Geometry: see drawing. Coordinates: mm, zero at the bounding-box minimum. A direction names the side the tool comes from. Give positions to 0.01 mm unless a question says otherwise; leave off trailing zeros. Write each loop counter-clockwise with the first axis right and the second up, starting at its lowest first coordinate (ties: lowest second). Pieces come first, ordered by that corner, then holes. Notation, with made-up numbers: (78.25, -3.75) -> (130.25, -3.75) arc R20 cw to (130.25, 35.25) -> close; hole circle Ø6 at (88, 88.5). An arc over 180 degrees is marked (long way). Answer as a JSON object with one key per item and string values. Group by question number.
Item 1: Pull-direction query (X, two-part tool) for the marked faces 1, 2, 3 and 4; classes: pulls with the +X half, pulls with the -X half, needs draft (parallel to the pull), parting line crosses it, or undercut.
Item 2: Ray query, probe 1 along Y at (x, z) = (8, 4.5) (1 decimal); probe 2 along Y at (x, z) = (8, 1.75) (1 decimal); probe 3 along Z at (x, y) = (9, 11.95) (1 decimal). Return the intervals inside material, ascending. Write a range as from..to.
Item 3: Access query for the marked faces 5, 6, 7 and 8. Directions: +Z, -Z, +X, -X, +Y, -Y. A direction counts if a zero-diameter tool reaches every point of the face in a straight line with its end or side. Return the directions, or none.
Item 4: Section query A-A on x = 9. Give the number of separate pieces and of enclosed holes in the cut face, plus the area to 3 significant figures.
Item 5: First-contact query: pin 1 Ø2.5 at (x, y) = (13.87, 11.81) entering from +Z; pin 2 Ø6 at (x, z) = (13.5, 14.5) entering from -Y (1 decimal); pin 3 Ø3 at (y, z) = (10.5, 9) entering from -X; pin 4 Ø1 at (x, y) = (12, 2.5) entering from +Z. Flat tips, straight axial feed; report the tip coordinate or a pass-through.
Item 6: Section query B-B on y = 9. Return the cut outline in (x, z).
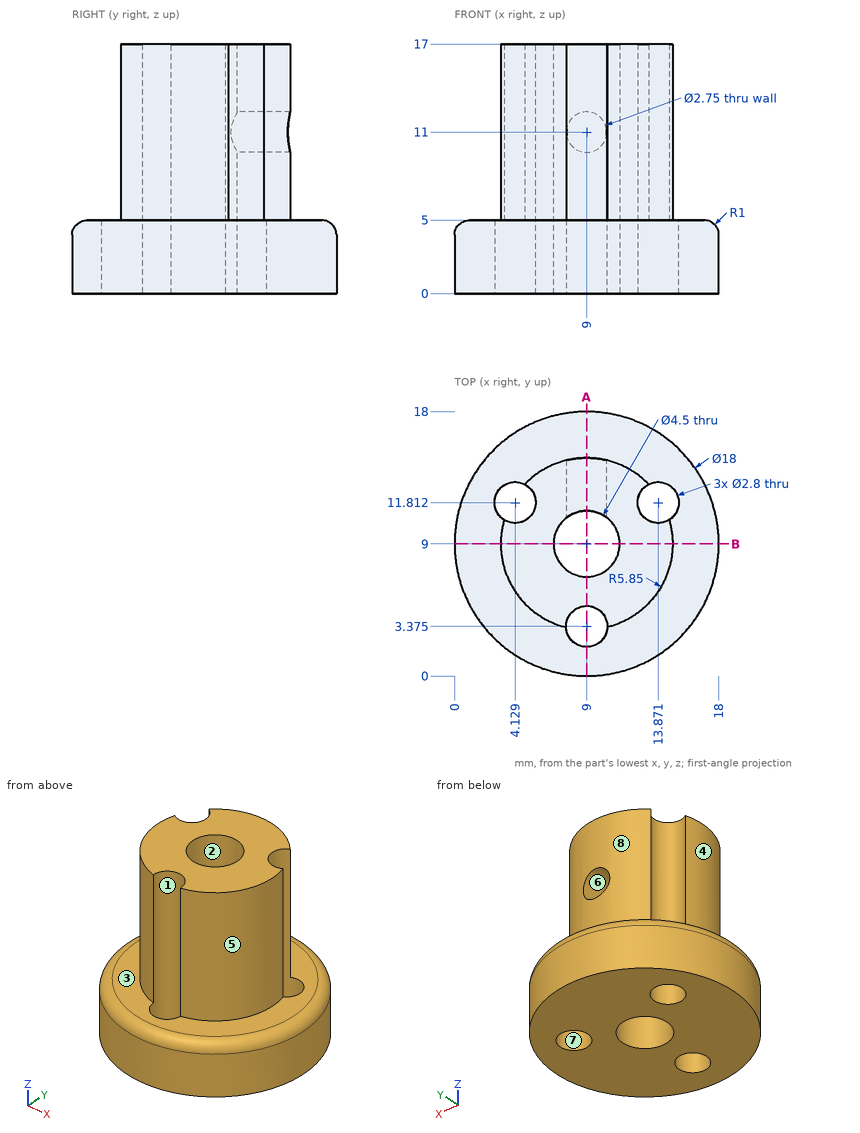
Worked answers:
{
 "1": {"face 1": "undercut", "face 2": "undercut", "face 3": "needs draft", "face 4": "pulls with the -X half"},
 "2": {"probe 1": "0.2..2.4, 4.4..7, 11..17.8", "probe 2": "0.1..2.4, 4.4..7, 11..17.9", "probe 3": "0..9.6, 12.4..17"},
 "3": {"face 5": "+Z, +X", "face 6": "+Y", "face 7": "+Z, -Z", "face 8": "+Z, +Y"},
 "4": {"separate pieces": "4", "enclosed holes": "0", "area": "110 mm^2"},
 "5": {"pin 1": "through", "pin 2": "y = 3.3", "pin 3": "x = 3.15", "pin 4": "z = 5"},
 "6": {"outline": "(0, 0) -> (6.75, 0) -> (6.75, 17) -> (3.15, 17) -> (3.15, 5) -> (1, 5) arc R1 ccw to (0, 4) -> close; (11.25, 0) -> (18, 0) -> (18, 4) arc R1 ccw to (17, 5) -> (14.85, 5) -> (14.85, 17) -> (11.25, 17) -> close"}
}
